```python
from build123d import *

# Parameters (mm, degrees)
ESBO_O1_R                = 7.5
RESSALTO_EXTRUS_O1_DEPTH = 60.825
CORTE_EXTRUS_O1_START    = -7.5
ESBO_O2_R                = 7.5
ESBO_O2_R_2              = 6.5
CORTE_EXTRUS_O1_DEPTH    = 7.5
CHANFRO1_SIZE            = 0.5


with BuildPart() as part:
    # Esboço1 → Ressalto-extrusão1 (new, symmetric)
    with BuildSketch(Plane.XY):
        with Locations(Location((0, 0, 0), (0, 0, 180))):
            Circle(ESBO_O1_R)
    extrude(amount=RESSALTO_EXTRUS_O1_DEPTH, both=True)

    # Esboço2 → Corte-extrusão1 (cut)
    with BuildSketch(Plane(origin=(0, 0, -60.825), x_dir=(-1, 0, 0), z_dir=(0, 0, -1)).offset(CORTE_EXTRUS_O1_START)):
        Circle(ESBO_O2_R)
        Circle(ESBO_O2_R_2, mode=Mode.SUBTRACT)
    corte_extrus_o1 = extrude(amount=CORTE_EXTRUS_O1_DEPTH, mode=Mode.SUBTRACT)

    # Esboço7 → Furo roscado de M6x1.01 (revolve, cut)
    with BuildSketch(Plane(origin=(0, 0, -60.825), x_dir=(0, 1, 0), z_dir=(1, 0, 0))):
        Polygon((0, 0), (0, 17), (2.5, 15.497848452), (2.5, 0), align=None)
    furo_roscado_de_m6x1_01 = revolve(axis=Axis((0, 0, -67.175), (0, 0, 1)), mode=Mode.SUBTRACT)

    # Espelhar1: Corte-extrusão1, Furo roscado de M6x1.01 across plane
    add(corte_extrus_o1.mirror(Plane.XY), mode=Mode.SUBTRACT)
    add(furo_roscado_de_m6x1_01.mirror(Plane.XY), mode=Mode.SUBTRACT)

    # Chanfro1
    chanfro1_edges = [part.edges().sort_by_distance(p)[0] for p in [
        (0, -2.5, -60.825),
        (6.5, 0, 60.825),
        (0, -2.5, 60.825),
        (6.5, 0, -60.825),
    ]]
    chamfer(chanfro1_edges, length=CHANFRO1_SIZE)


solid = part.part
```
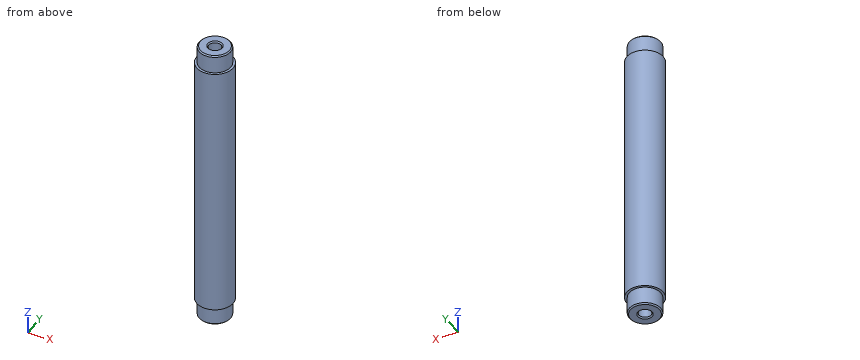
CAD build for the part. Positions are in the model's coordinates, mm. Coordinates: 2 decimals unless noted, no trailing zeros. Write each loop counter-clockwise with the first axis right and the second up, starting at its lowest first coordinate (ties: lowest second). Pieces come first, ordered by that corner, then holes. Notation, with made-up numbers: (56, 23) -> (94, 23) arc R24 ccw to (94, 58) -> close; hole circle Ø9 at (26, -39). An arc over 180 degrees is marked (long way). Return JSON: item names as keys, results as strings. Group by question number.
Q1. Cut at A-A, the plane z = 48. Give the cut face in (x, y).
Q2. Cut at B-B, the plane z = -36. Give the cut face in (x, y), then the cut area to 3 significant figures.
Q3. Flat gauge pins, fed straight in: pin 1 (3 mm diameter, centred on x = 0, y = 0, fed in from -Z); pin 2 (8 mm diameter, centred on x = -4.5, z = -12, fed in from -Y); pin 3 (4 mm diameter, centred on y = -6, z = 23, fed in from +X). Where does each tip first touch, or does it go through?
Q4. Drill centre lines: line 1 (Y direction, x = 0, z = 52); line 2 (Y direction, x = 0, z = 56.5); line 3 (Z direction, x = -6, y = 0.25). Where is each one in solid material? Low to high.
Returned:
{
 "1": {"outline": "circle Ø15 at (0, 0); hole circle Ø5 at (0, 0)"},
 "2": {"outline": "circle Ø15 at (0, 0)", "area": "177 mm2"},
 "3": {"pin 1": "stops at z = -44.73", "pin 2": "stops at y = -7.48", "pin 3": "stops at x = 6.34"},
 "4": {"line 1": "y = -7.5 to -2.5, 2.5 to 7.5", "line 2": "y = -6.5 to -2.5, 2.5 to 6.5", "line 3": "z = -60.82 to 60.82"}
}
